CAD build for the part. Positions are in the model's coordinates, mm. A direction names the side the tool comes from. Coordinates: 2 decimals unless noted, no trailing zeros. Loops run counter-clockwise (first coordinate to the right, second up) from the corner with the lowest first, then second, coordinate; pieces in that order, holes last.
1) Which spindle directions (+Z, -Z, +X, -X, +Y, -Y) get a long thin tool onto all of the face, cutting with end or side? Do faces 4 (the cylindrical face through (30.775, 267.336, 1.479)), 5 (the flat face through (10.91, 275.62, 1.48)). Say none if no direction does.
2) Two-plate mould, pull along Y, no slides. Class faces 1 (the flat face through (24, 273.129, 1)), 2 (the flat face through (20.216, 266, 1)), 3 (the flat face through (10.91, 269.62, 1.48)): +Y half, -Y half, draft (parallel to the pull), parting line (faces both ways), or undercut.
3) Saw through at B-B, the plane z = 1.1. Give the number of separate pieces and of enclosed holes in the cut face, and give its area (3 significant figures).
4) Wall check: line 1 along Y through (x, z) = (17, 2.55); line 2 along X through (y, z) = (287, 0.65); line 3 along X through (y, z) = (285.5, 2.15). Give the ranges that are in metal, low to high.
5) Pin check, flat tips, straight feed: pin 1 Ø1 at (y, z) = (281, 1) entering from -X; pin 2 Ø1.5 at (y, z) = (286, 2.5) entering from +X; pin 3 Ø0.6 at (y, z) = (266, 1) entering from +X. Stop position of each tip, or through.
6) Saw through at D-D, the plane y = 283.5. Write the cut outline in (x, z).
7) Saw through at A-A, the plane x = 17. Write the cut outline in (y, z).
8) Saw through at C-C, the plane x = 26.5. Write the cut outline in (y, z), and give its area (3 significant figures).
```python
from build123d import *

# Parameters (mm, degrees)
MODEL_R                 = 1.5
SALIENTE_EXTRUIR1_DEPTH = 3


with BuildPart() as part:
    # Model → Saliente-Extruir1 (new body)
    with BuildSketch(Plane.XY):
        with BuildLine():
            Line((10.417346401, 265.129037091), (11.417346401, 266.129037091))
            Line((11.417346401, 266.129037091), (10.417346401, 267.129037091))
            Line((10.417346401, 267.129037091), (11.417346401, 268.129037091))
            Line((11.417346401, 268.129037091), (10.417346401, 269.129037091))
            Line((10.417346401, 269.129037091), (11.417346401, 270.129037091))
            Line((11.417346401, 270.129037091), (10.417346401, 271.129037091))
            Line((10.417346401, 271.129037091), (11.417346401, 272.129037091))
            Line((11.417346401, 272.129037091), (10.417346401, 273.129037091))
            Line((10.417346401, 273.129037091), (11.417346401, 274.129037091))
            Line((11.417346401, 274.129037091), (10.417346401, 275.129037091))
            Line((10.417346401, 275.129037091), (11.417346401, 276.129037091))
            Line((11.417346401, 276.129037091), (10.417346401, 277.129037091))
            Line((10.417346401, 277.129037091), (11.417346401, 278.129037091))
            Line((11.417346401, 278.129037091), (10.417346401, 279.129037091))
            Line((10.417346401, 279.129037091), (11.417346401, 280.129037091))
            Line((11.417346401, 280.129037091), (10.417346401, 281.129037091))
            Line((10.417346401, 281.129037091), (11.417346401, 282.129037091))
            Line((11.417346401, 282.129037091), (10.417346401, 283.129037091))
            Line((10.417346401, 283.129037091), (11.417346401, 284.129037091))
            Line((11.417346401, 284.129037091), (10.417346401, 285.129037091))
            Line((10.417346401, 285.129037091), (11.417346401, 286.129037091))
            Line((11.417346401, 286.129037091), (10.417346401, 287.129037091))
            Line((10.417346401, 287.129037091), (11.417346401, 288.129037091))
            Line((11.417346401, 288.129037091), (10.417346401, 289.129037091))
            Line((10.417346401, 289.129037091), (11.417346401, 290.129037091))
            Line((11.417346401, 290.129037091), (10.417346401, 291.129037091))
            Line((10.417346401, 291.129037091), (15.917346401, 291.129037091))
            ThreePointArc((15.917346401, 291.129037091), (19.099326917, 289.811017606), (20.417346401, 286.629037091))
            Line((20.417346401, 286.629037091), (20.417346401, 273.129037091))
            Line((20.417346401, 273.129037091), (27.417346401, 273.129037091))
            ThreePointArc((27.417346401, 273.129037091), (30.267267915, 272.111557351), (31.828417252, 269.51923592))
            ThreePointArc((31.828417252, 269.51923592), (31.838364225, 268.980221543), (31.657098407, 268.472502977))
            Line((31.657098407, 268.472502977), (31.314460718, 267.879037091))
            ThreePointArc((31.314460718, 267.879037091), (30.765422613, 267.329998985), (30.015422613, 267.129037091))
            Line((30.015422613, 267.129037091), (21.515422613, 267.129037091))
            ThreePointArc((21.515422613, 267.129037091), (20.845676718, 266.971214589), (20.316865454, 266.530957674))
            ThreePointArc((20.316865454, 266.530957674), (20.242169616, 266.388811129), (20.216384507, 266.23031748))
            Line((20.216384507, 266.23031748), (20.216384507, 265.027756703))
            ThreePointArc((20.216384507, 265.027756703), (20.190599398, 264.869263053), (20.11590356, 264.727116508))
            ThreePointArc((20.11590356, 264.727116508), (19.587092296, 264.286859593), (18.917346401, 264.129037091))
            Line((18.917346401, 264.129037091), (11.417346401, 264.129037091))
            Line((11.417346401, 264.129037091), (10.417346401, 265.129037091))
        make_face()
        with Locations((15.917346401, 268.629037091)):
            Circle(MODEL_R, mode=Mode.SUBTRACT)
        with Locations((15.917346401, 277.629037091)):
            Circle(MODEL_R, mode=Mode.SUBTRACT)
        with Locations((15.917346401, 286.629037091)):
            Circle(MODEL_R, mode=Mode.SUBTRACT)
    extrude(amount=SALIENTE_EXTRUIR1_DEPTH)


solid = part.part
```
Data:
1. face 4: +Z, -Z, +X, -Y
1. face 5: +Z, -Z, -X
2. face 1: +Y half
2. face 2: draft
2. face 3: undercut
3. separate pieces: 1
3. enclosed holes: 3
3. area: 294 mm2
4. line 1: y = 264.13 to 267.59, 269.67 to 276.59, 278.67 to 285.59, 287.67 to 291
4. line 2: x = 10.55 to 14.46, 17.37 to 20.4
4. line 3: x = 10.79 to 14.93, 16.9 to 20.42
5. pin 1: stops at x = 10.42
5. pin 2: stops at x = 20.42
5. pin 3: stops at x = 20.22
6. outline: (10.79, 0) - (20.42, 0) - (20.42, 3) - (10.79, 3) - close
7. outline: (264.13, 0) - (267.59, 0) - (267.59, 3) - (264.13, 3) - close; (269.67, 0) - (276.59, 0) - (276.59, 3) - (269.67, 3) - close; (278.67, 0) - (285.59, 0) - (285.59, 3) - (278.67, 3) - close; (287.67, 0) - (291, 0) - (291, 3) - (287.67, 3) - close
8. outline: (267.13, 0) - (273.13, 0) - (273.13, 3) - (267.13, 3) - close
8. area: 18.0 mm2
